from build123d import *

# Parameters (mm, degrees)
F2_R     = 1.27
F3_DEPTH = 5.08


# Not quite as in the source:
# - a feature names something its author has since deleted; it is built from what else it names


with BuildPart() as f1:
    # F0 (on Front) → F1 (revolve)
    with BuildSketch(Plane.XZ):
        with BuildLine():
            Line((0, 76.2), (0, 0))
            Line((0, 0), (3.683, 0))
            Line((3.683, 0), (3.683, 50.5892820656))
            Line((3.683, 50.5892820656), (3.683, 75.4657239321))
            add(Edge.make_bspline(
                [(3.683, 75.4657239321), (3.9001026563, 75.5844257372), (4.117282526, 75.702956664), (4.3289103642, 75.8188781839)],
                knots=[0, 0, 0, 0, 0.0367930761, 0.0367930761, 0.0367930761, 0.0367930761], degree=3))
            Line((4.3289103642, 75.8188781839), (4.7080438681, 77.083454169))
            Line((4.7080438681, 77.083454169), (5.4083663136, 77.7371979129))
            Line((5.4083663136, 77.7371979129), (5.8970035864, 78.2753947108))
            add(Edge.make_bspline(
                [(5.8970035864, 78.2753947108), (5.4557518487, 78.5243036944), (3.6824791799, 79.0277734306), (3.8959075155, 80.928711884), (2.7015379677, 83.0135115397), (2.599091359, 84.685822435), (2.3724716532, 85.744447935), (2.2606033154, 86.2670275395)],
                knots=[0.4795528936, 0.4795528936, 0.4795528936, 0.4795528936, 0.5884154591, 0.6871467774, 0.8044356188, 0.9034623818, 1, 1, 1, 1], degree=3))
            Line((2.2606033154, 86.2670275395), (0, 86.2670275395))
            Line((0, 86.2670275395), (0, 85.744447935))
            Line((0, 85.744447935), (0, 76.2))
        make_face()
    revolve(axis=Axis((0, 0, 38.1), (0, 0, 1)))

    # F2 (on face) → F3 (cut)
    with BuildSketch(Plane.XY.offset(86.2670275395)):
        Circle(F2_R)
    extrude(amount=-F3_DEPTH, mode=Mode.SUBTRACT)


solid = f1.part
Input: part model. Units: mm. Frame: model coordinates. A direction names the side the tool comes from. Coordinates: 2 decimals unless noted, no trailing zeros. Write each loop counter-clockwise with the first axis right and the second up, starting at its lowest first coordinate (ties: lowest second). Pieces come first, ordered by that corner, then holes. Notation, with made-up numbers: M 12.5,69.5 L 26.5,69.5 A24 ccw 26.5,104.5 Z; hole C -35,10.5 d2. An arc over 180 degrees is marked long. Answer as a JSON object with one key per item and string values. Group by question number.
(1) Section A-A on z = 37. Output: boundary loops of the cut face in (x, y), plus the area to 3 significant figures.
(2) Mould query, pull axis X, two halves, no side actions, for faces 1 (the face through (0, -1.5, 86.267)), 2 (the face through (0, 0, 81.187)), 3 (the face through (1.699, -3.267, 38.261)). Classes: pulls with the +X half, pulls with the -X half, needs draft (parallel to the pull), parting line crosses it, or undercut.
(3) Ray query, line 1 along Z through (x, y) = (-0.5, 0.5); line 2 along Y through (x, z) = (0, 83.35); line 3 along Y through (x, z) = (0, 83.7). Return the intervals inside material, ascending. Write a range as [from, to].
(4) Contact query for flat-ended pins moving along their axis: P1, Ø2, axis at x = 0.5, y = -0.5, coming from the +Z side; P2, Ø2, axis at y = 2.5, z = 58, coming from the -X side; P3, Ø4, axis at y = 0.5, z = 76, coming from the +X side; P4, Ø2, axis at x = 3.5, z = 64, coming from the +Y side. Output: stop coordinate, or through.
(5) Set-up query: faces 4 (the face through (-0.17, 1.26, 83.76)), 5 (the face through (0, 0, 0)). Return all of +Z, -Z, +X, -X, +Y, -Y with unobstructed straight access to the full face (end or side cutting, diameter ignored); none if empty.
Result set:
{
 "1": {"outline": "C 0,0 d7.37", "area": "42.6 mm2"},
 "2": {"face 1": "needs draft", "face 2": "undercut", "face 3": "parting line crosses it"},
 "3": {"line 1": "z = [0, 81.19]", "line 2": "y = [-2.77, -1.27], [1.27, 2.77]", "line 3": "y = [-2.69, -1.27], [1.27, 2.69]"},
 "4": {"P1": "stops at z = 86.27", "P2": "stops at x = -3.36", "P3": "stops at x = 5.63", "P4": "stops at y = 2.7"},
 "5": {"face 4": "+Z", "face 5": "-Z, +X, -X, +Y, -Y"}
}
